Build history of the part. All positions in model axes, mm. Face numbers are marked on the shaded views. Coordinates: 2 decimals unless noted, no trailing zeros. Write each loop counter-clockwise with the first axis right and the second up, starting at its lowest first coordinate (ties: lowest second). Pieces come first, ordered by that corner, then holes. Notation, with made-up numbers: M -23.75,-40 L 17.25,-40 A26 ccw 17.25,-26 Z; hole C 10,65.5 d10. An arc over 180 degrees is marked long. Use CSV: the item, a comma, the result in double quotes. Start each with the question number.
```python
from build123d import *

# Parameters (mm, degrees)
SKETCH1_W            = 25.019
SKETCH1_H            = 19.05
BOSS_EXTRUDE1_DEPTH  = 8.001
SKETCH2_W            = 0.508
SKETCH2_H            = 0.254
BOSS_EXTRUDE2_DEPTH  = 4.064
LPATTERN1_COUNT      = 5
LPATTERN1_PITCH      = 2.54
LPATTERN1_COUNT_DIR2 = 2
LPATTERN1_PITCH_DIR2 = 15.24
LPATTERN2_COUNT      = 5
LPATTERN2_PITCH      = 2.54
LPATTERN2_COUNT_DIR2 = 2
LPATTERN2_PITCH_DIR2 = 15.24
SKETCH4_R            = 0.8382
CUT_EXTRUDE1_DEPTH   = 0.0254
LPATTERN3_COUNT      = 2
LPATTERN3_PITCH      = 12.7


with BuildPart() as part:
    # Sketch1 → Boss-Extrude1 (new body)
    with BuildSketch(Plane.XY):
        Rectangle(SKETCH1_W, SKETCH1_H)
    extrude(amount=BOSS_EXTRUDE1_DEPTH)

    # Sketch2 → Boss-Extrude2 (add)
    with BuildSketch(Plane(origin=(0, 0, 0), x_dir=(-1, 0, 0), z_dir=(0, 0, -1))):
        with Locations((0, 7.62)):
            Rectangle(SKETCH2_W, SKETCH2_H)
    boss_extrude2 = extrude(amount=BOSS_EXTRUDE2_DEPTH)

    # LPattern1: Boss-Extrude2 5 × 2
    with Locations(*[(-i * LPATTERN1_PITCH, -j * LPATTERN1_PITCH_DIR2, 0) for i in range(LPATTERN1_COUNT) for j in range(LPATTERN1_COUNT_DIR2) if (i, j) != (0, 0)]):
        add(boss_extrude2)

    # LPattern2: Boss-Extrude2 5 × 2
    with Locations(*[(i * LPATTERN2_PITCH, -j * LPATTERN2_PITCH_DIR2, 0) for i in range(LPATTERN2_COUNT) for j in range(LPATTERN2_COUNT_DIR2) if (i, j) != (0, 0)]):
        add(boss_extrude2)

    # Sketch4 → Cut-Extrude1 (cut)
    with BuildSketch(Plane.XY.offset(8.001)):
        with Locations((-1.5875, -6.2738)):
            Circle(SKETCH4_R)
        Polygon((-9.556202543, 0), (-9.048202543, 0.508), (-3.651797457, 0.508), (-3.143797457, 0), (-3.651797457, -0.508), (-9.048202543, -0.508), align=None)
        with BuildLine():
            Line((-9.788412788, 0.127), (-9.348244077, 0.567168711))
            Line((-9.348244077, 0.567168711), (-8.428428025, 7.112))
            Line((-8.428428025, 7.112), (-9.012815176, 7.112))
            ThreePointArc((-9.012815176, 7.112), (-9.346093162, 6.987392467), (-9.515871354, 6.674699935))
            Line((-9.515871354, 6.674699935), (-10.436090569, 0.127))
            Line((-10.436090569, 0.127), (-9.788412788, 0.127))
        make_face()
        Polygon((-5.350473584, 7.112), (-8.171931821, 7.112), (-8.313331692, 6.105887642), (-5.491873454, 6.105887642), (-2.670415217, 6.105887642), (-2.529015346, 7.112), align=None)
        with BuildLine():
            Line((-2.085422571, 0.127), (-2.911587212, 0.127))
            Line((-2.911587212, 0.127), (-3.211979491, 0.427392279))
            Line((-3.211979491, 0.427392279), (-2.272519143, 7.112))
            Line((-2.272519143, 7.112), (-1.688131992, 7.112))
            ThreePointArc((-1.688131992, 7.112), (-1.304739525, 6.937277987), (-1.185075813, 6.533300065))
            Line((-1.185075813, 6.533300065), (-2.085422571, 0.127))
        make_face()
        with BuildLine():
            Line((-3.544395336, -7.112), (-4.271571975, -7.112))
            Line((-4.271571975, -7.112), (-3.351755923, -0.567168711))
            Line((-3.351755923, -0.567168711), (-2.911587212, -0.127))
            Line((-2.911587212, -0.127), (-2.121119943, -0.127))
            Line((-2.121119943, -0.127), (-3.041339158, -6.674699935))
            ThreePointArc((-3.041339158, -6.674699935), (-3.21111735, -6.987392467), (-3.544395336, -7.112))
        make_face()
        with BuildLine():
            Line((-10.471787941, -0.127), (-9.788412788, -0.127))
            Line((-9.788412788, -0.127), (-9.488020509, -0.427392279))
            Line((-9.488020509, -0.427392279), (-10.427480857, -7.112))
            Line((-10.427480857, -7.112), (-10.86907852, -7.112))
            ThreePointArc((-10.86907852, -7.112), (-11.252470987, -6.937277987), (-11.372134699, -6.533300065))
            Line((-11.372134699, -6.533300065), (-10.471787941, -0.127))
        make_face()
        Polygon((-7.208126546, -6.105887642), (-10.029584783, -6.105887642), (-10.170984654, -7.112), (-7.349526416, -7.112), (-4.528068179, -7.112), (-4.386668308, -6.105887642), align=None)
    cut_extrude1 = extrude(amount=-CUT_EXTRUDE1_DEPTH, mode=Mode.SUBTRACT)

    # LPattern3: Cut-Extrude1 ×2
    with Locations(*[(i * LPATTERN3_PITCH, 0, 0) for i in range(1, LPATTERN3_COUNT)]):
        add(cut_extrude1, mode=Mode.SUBTRACT)


solid = part.part
```
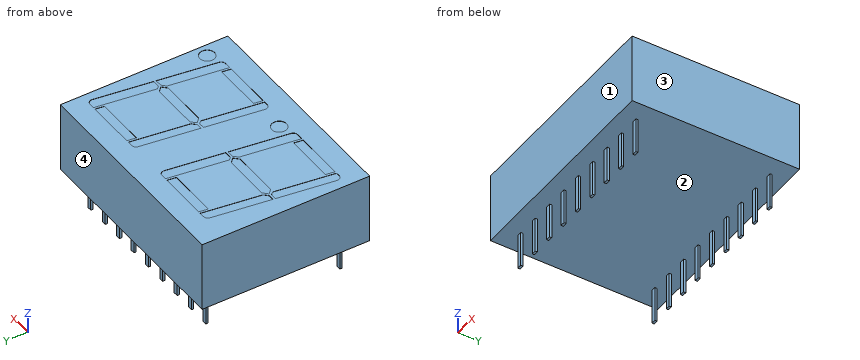
1. Slice it at D-D (x = 1). List the corners of the cut face in (y, z) (3 decimals).
2. Slice it at B-B (z = -1.5). Count the separate pieces of the cut face and the enclosed holes in it, and give its area (3 significant figures).
3. Drill centre lines: line 1 along Y through (x, z) = (0, -1); line 2 along Z through (x, y) = (-7.25, -5.25). Where is each one in solid material? Low to high. Write a range as from..to.
4. Flat gauge pins, fed straight in: pin 1 (1.5 mm diameter, centred on x = -9, z = -2, fed in from +Y); pin 2 (1.5 mm diameter, centred on x = -9, y = 4.5, fed in from -Z). Where does each tip first touch, or does it go through?
5. Pull direction Y, two halves, no side cores. Call the marked faces 1, 2, 3 and 4: pulls with the +Y half, pulls with the -Y half, needs draft (parallel to the pull), parting line crosses it, or undercut.
6. Slice it at A-A (x = -6.25). List the corners of the cut face in (y, z) (3 decimals).
Established:
1,outline,"M -9.525,0 L 9.525,0 L 9.525,8.001 L -9.525,8.001 Z"
2,separate pieces,"18"
2,enclosed holes,"0"
2,area,"2.32 mm2"
3,line 1,"y = -7.75..-7.49, 7.49..7.75"
3,line 2,"z = 0..8"
4,pin 1,"passes through"
4,pin 2,"stops at z = 0"
5,face 1,"pulls with the -Y half"
5,face 2,"undercut"
5,face 3,"needs draft"
5,face 4,"pulls with the +Y half"
6,outline,"M -9.525,0 L 9.525,0 L 9.525,8.001 L 7.112,8.001 L 7.112,7.976 L 6.106,7.976 L 6.106,8.001 L 0.508,8.001 L 0.508,7.976 L -0.508,7.976 L -0.508,8.001 L -6.106,8.001 L -6.106,7.976 L -7.112,7.976 L -7.112,8.001 L -9.525,8.001 Z"
